For this review, take the finished solid that the model builds, in its own axes (mm). A direction names the side the tool comes from. Coordinates: 2 decimals unless noted, no trailing zeros. Write each loop counter-clockwise with the first axis right and the second up, starting at its lowest first coordinate (ties: lowest second). Pieces come first, ordered by that corner, then holes. Notation, with made-up numbers: (25.25, 10) -> (33.25, 10) arc R28 cw to (33.25, 36) -> close; hole circle Ø10 at (57.25, -4.75). An arc over 180 degrees is marked (long way). Put each result on its own line as item: value. Start each with the question number.
Item 1: For faces 1 (the cylindrical face through (-4.507, 0.481, 81.526)), 2 (the cylindrical face through (0.1, -4.5, 93)), list the 3-axis set-ups (+Z, -Z, +X, -X, +Y, -Y) from which the entire face can be reached by the end or side of a thin tool; tool diameter is ignored.
Item 2: Consider section B-B on z = 115. Give the boundary of the cut face in (x, y), and give its area (3 significant figures).
Item 3: Consider section A-A on z = 80. Give the boundary of the cut face in (x, y).
Item 4: Insertion check: P1, Ø1.9, axis at y = 0, z = 40, coming from the -X side. The pin has a flat end and moves straight along its axis. Give the tip position at first contact, or say it passes through.
Item 5: The part is to be moulded in two halves that separate along Y. For faces 3 (the flat face through (0, 5, 59)), 4 (the cylindrical face through (-4.51, 1.08, 23.82)), 5 (the flat face through (4, 0, 59)), 6 (the cylindrical face through (0.1, -4.5, 12)), say which applies: +Y half, -Y half, draft (parallel to the pull), parting line (faces both ways), or undercut.
Item 6: To check wall thickness, follow L1, parallel to Y at x = 2, z = 79; L2, parallel to Y at x = 4.2, z = 25. State the ranges of each line that lie inside material, in increasing order.
```python
from build123d import *

# Parameters (mm, degrees)
SKETCH_1_W          = 10
SKETCH_1_H          = 10
SKETCH_1_W_2        = 8
SKETCH_1_H_2        = 8
EXTRUDE_1_DEPTH     = 120
SKETCH_2_R          = 3
CUT_EXTRUDE_1_DEPTH = 121.519707932
SKETCH_3_R          = 3
CUT_EXTRUDE_2_DEPTH = 10
SKETCH_4_R          = 1.6
CUT_EXTRUDE_3_DEPTH = 10
SKETCH_5_R          = 1.6
CUT_EXTRUDE_4_DEPTH = 121.519707932
SKETCH_6_R          = 3
CUT_EXTRUDE_5_DEPTH = 2
SKETCH_7_R          = 1.6
CUT_EXTRUDE_6_DEPTH = 121.519707932


with BuildPart() as part:
    # ｽｹｯﾁ1 → ﾎﾞｽ - 押し出し1 (new body)
    with BuildSketch(Plane.XY):
        Rectangle(SKETCH_1_W, SKETCH_1_H)
        Rectangle(SKETCH_1_W_2, SKETCH_1_H_2, mode=Mode.SUBTRACT)
    extrude(amount=EXTRUDE_1_DEPTH)

    # ｽｹｯﾁ2 → ｶｯﾄ - 押し出し1 (cut, through all)
    with BuildSketch(Plane.ZY.offset(5)):
        with Locations((5, 0)):
            Circle(SKETCH_2_R)
        with Locations((115, 0)):
            Circle(SKETCH_2_R)
    extrude(amount=-CUT_EXTRUDE_1_DEPTH, mode=Mode.SUBTRACT)

    # ｽｹｯﾁ3 → ｶｯﾄ - 押し出し2 (cut)
    with BuildSketch(Plane(origin=(0, 5, 0), x_dir=(1, 0, 0), z_dir=(0, 1, 0))):
        with Locations(Location((0, -105, 0), (0, 0, 270))):
            Circle(SKETCH_3_R)
        with Locations(Location((0, -15, 0), (0, 0, 270))):
            Circle(SKETCH_3_R)
    extrude(amount=-CUT_EXTRUDE_2_DEPTH, mode=Mode.SUBTRACT)

    # ｽｹｯﾁ4 → ｶｯﾄ - 押し出し3 (cut)
    with BuildSketch(Plane(origin=(0, 5, 0), x_dir=(1, 0, 0), z_dir=(0, 1, 0))):
        with Locations(Location((0, -30, 0), (0, 0, 270))):
            Circle(SKETCH_4_R)
        with Locations(Location((0, -90, 0), (0, 0, 270))):
            Circle(SKETCH_4_R)
    extrude(amount=-CUT_EXTRUDE_3_DEPTH, mode=Mode.SUBTRACT)

    # ｽｹｯﾁ5 → ｶｯﾄ - 押し出し4 (cut, through all)
    with BuildSketch(Plane.ZY.offset(5)):
        with Locations((25, 0)):
            Circle(SKETCH_5_R)
        with Locations((95, 0)):
            Circle(SKETCH_5_R)
    extrude(amount=-CUT_EXTRUDE_4_DEPTH, mode=Mode.SUBTRACT)

    # ｽｹｯﾁ6 → ｶｯﾄ - 押し出し5 (cut)
    with BuildSketch(Plane(origin=(0, -5, 0), x_dir=(-1, 0, 0), z_dir=(0, -1, 0))):
        with Locations(Location((0, -30, 0), (0, 0, 90))):
            Circle(SKETCH_6_R)
        with Locations(Location((0, -90, 0), (0, 0, 90))):
            Circle(SKETCH_6_R)
    extrude(amount=-CUT_EXTRUDE_5_DEPTH, mode=Mode.SUBTRACT)

    # ｽｹｯﾁ7 → ｶｯﾄ - 押し出し6 (cut, through all)
    with BuildSketch(Plane.ZY.offset(5)):
        with Locations((80, 0)):
            Circle(SKETCH_7_R)
        with Locations((40, 0)):
            Circle(SKETCH_7_R)
    extrude(amount=-CUT_EXTRUDE_6_DEPTH, mode=Mode.SUBTRACT)


solid = part.part
```
Return value:
1. face 1: +X, -X
1. face 2: -Y
2. outline: (-5, -5) -> (5, -5) -> (5, -3) -> (4, -3) -> (4, -4) -> (-4, -4) -> (-4, -3) -> (-5, -3) -> close; (-5, 3) -> (-4, 3) -> (-4, 4) -> (4, 4) -> (4, 3) -> (5, 3) -> (5, 5) -> (-5, 5) -> close
2. area: 24.0 mm^2
3. outline: (-5, -5) -> (5, -5) -> (5, -1.6) -> (4, -1.6) -> (4, -4) -> (-4, -4) -> (-4, -1.6) -> (-5, -1.6) -> close; (-5, 1.6) -> (-4, 1.6) -> (-4, 4) -> (4, 4) -> (4, 1.6) -> (5, 1.6) -> (5, 5) -> (-5, 5) -> close
4. P1: through
5. face 3: +Y half
5. face 4: undercut
5. face 5: undercut
5. face 6: draft
6. L1: -5 to -4, 4 to 5
6. L2: -5 to -1.6, 1.6 to 5
